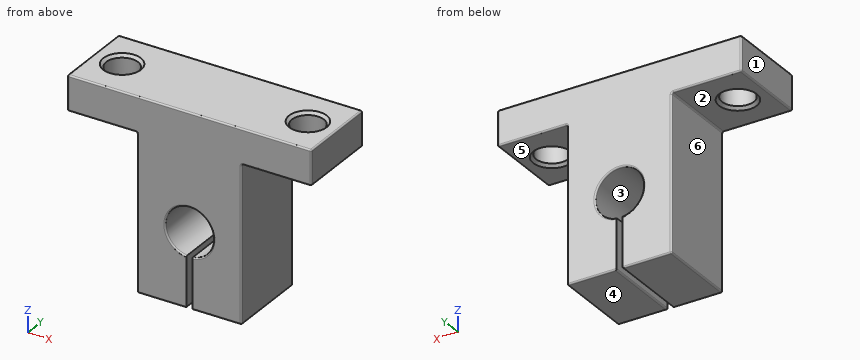
from build123d import *

# Parameters (mm, degrees)
BOSS_EXTRUDE1_DEPTH      = 7
BOSS_EXTRUDE1_DEPTH_BACK = 7
CUT_EXTRUDE1_REACH       = 34.8
SKETCH2_R                = 2.75
FILLET1_R                = 0.25
CHAMFER1_SIZE            = 0.5


with BuildPart() as part:
    # Sketch1 → Boss-Extrude1 (new body, two sides)
    with BuildSketch(Plane(origin=(0, 0, 0), x_dir=(1, 0, 0), z_dir=(0, 1, 0))) as boss_extrude1_sk:
        with BuildLine():
            Line((-21, 6), (-21, 0))
            Line((-21, 0), (0, 0))
            Line((0, 0), (0, 15.85))
            ThreePointArc((0, 15.85), (-4.142435459, 19.749543473), (-0.5, 24.119769411))
            Line((-0.5, 24.119769411), (-0.5, 32.8))
            Line((-0.5, 32.8), (-9, 32.8))
            Line((-9, 32.8), (-9, 6))
            Line((-9, 6), (-21, 6))
        make_face()
        with BuildLine():
            Line((0, 15.85), (0, 0))
            Line((0, 0), (21, 0))
            Line((21, 0), (21, 6))
            Line((21, 6), (9, 6))
            Line((9, 6), (9, 32.8))
            Line((9, 32.8), (0.5, 32.8))
            Line((0.5, 32.8), (0.5, 24.119769411))
            ThreePointArc((0.5, 24.119769411), (3.106243712, 22.752044694), (4.15, 20))
            ThreePointArc((4.15, 20), (2.934493142, 17.065506858), (0, 15.85))
        make_face()
    extrude(amount=BOSS_EXTRUDE1_DEPTH)
    extrude(boss_extrude1_sk.sketch, amount=-BOSS_EXTRUDE1_DEPTH_BACK)

    # Sketch2 → Cut-Extrude1 (cut, up to next)
    with BuildSketch(Plane.XY, mode=Mode.PRIVATE) as cut_extrude1_sk1:
        with Locations((-16, 0)):
            Circle(SKETCH2_R)
    cut_extrude1_tool1 = extrude(cut_extrude1_sk1.sketch, amount=-CUT_EXTRUDE1_REACH, mode=Mode.PRIVATE) & part.part
    add(cut_extrude1_tool1.solids().sort_by_distance((-16, 0, 0))[0], mode=Mode.SUBTRACT)
    # Sketch2 → Cut-Extrude1 (cut, up to next)
    with BuildSketch(Plane.XY, mode=Mode.PRIVATE) as cut_extrude1_sk2:
        with Locations((16, 0)):
            Circle(SKETCH2_R)
    cut_extrude1_tool2 = extrude(cut_extrude1_sk2.sketch, amount=-CUT_EXTRUDE1_REACH, mode=Mode.PRIVATE) & part.part
    add(cut_extrude1_tool2.solids().sort_by_distance((16, 0, 0))[0], mode=Mode.SUBTRACT)

    # Fillet1
    fillet1_edges = [part.edges().sort_by_distance(p)[0] for p in [
        (-4.75, -7, -32.8),
        (-9, -7, -19.4),
        (0.5, 0, -32.8),
        (9, 0, -32.8),
        (9, 0, -6),
        (21, 0, -6),
        (21, 0, 0),
        (-21, 0, 0),
        (-21, 0, -6),
        (-9, 0, -6),
        (-9, 0, -32.8),
        (-0.5, 0, -32.8),
        (-15, -7, -6),
        (-21, -7, -3),
        (0, 7, -15.85),
        (-4.75, 7, -32.8),
        (-21, 7, -3),
        (0, -7, 0),
        (15, 7, -6),
        (9, 7, -19.4),
        (4.75, 7, -32.8),
        (-9, 7, -19.4),
        (-15, 7, -6),
        (0, 7, 0),
        (21, 7, -3),
        (21, -7, -3),
        (15, -7, -6),
        (0, -7, -15.85),
        (9, -7, -19.4),
        (4.75, -7, -32.8),
    ]]
    fillet(fillet1_edges, radius=FILLET1_R)

    # Chamfer1
    chamfer1_edges = [part.edges().sort_by_distance(p)[0] for p in [
        (-18.75, 0, -6),
        (-18.75, 0, 0),
        (13.25, 0, 0),
        (13.25, 0, -6),
    ]]
    chamfer(chamfer1_edges, length=CHAMFER1_SIZE)


solid = part.part
Read the model definition and answer for the solid it produces. Units are mm, in the model's axes. Face numbers are marked on the shaded views. A direction names the side the tool comes from. Give positions to 0.01 mm unless a question says otherwise; leave off trailing zeros. Loops run counter-clockwise (first coordinate to the right, second up) from the corner with the lowest first, then second, coordinate; pieces in that order, holes last. Notation, with made-up numbers: M 64.5,35.5 L 96.5,35.5 A26 ccw 96.5,51.5 Z; hole C 41.25,20.25 d5. An arc over 180 degrees is marked long. Write each question's results on one line, items separated by ' | '.
1. Section A-A on x = -16 is taken. Give the vertices of the cut face in (y, z), plus the area to 3 significant figures.
Values:
outline: M -7,-5.75 A0.25 ccw -6.75,-6 L -3.25,-6 L -2.75,-5.5 L -2.75,-0.5 L -3.25,0 L -6.75,0 A0.25 ccw -7,-0.25 Z; M 2.75,-5.5 L 3.25,-6 L 6.75,-6 A0.25 ccw 7,-5.75 L 7,-0.25 A0.25 ccw 6.75,0 L 3.25,0 L 2.75,-0.5 Z | area: 50.4 mm^2
2. Section C-C on z = -15 is taken. Give the vertices of the cut face in (x, y), plus the area to 3 significant figures.
Values:
outline: M -9,-6.75 A0.25 ccw -8.75,-7 L 8.75,-7 A0.25 ccw 9,-6.75 L 9,6.75 A0.25 ccw 8.75,7 L -8.75,7 A0.25 ccw -9,6.75 Z | area: 252 mm^2
3. Section B-B on y = -5.5 is taken. Give the vertices of the cut face in (x, z).
Values:
outline: M -21,-5.75 A0.25 ccw -20.75,-6 L -9.25,-6 A0.25 cw -9,-6.25 L -9,-32.55 A0.25 ccw -8.75,-32.8 L -0.75,-32.8 A0.25 ccw -0.5,-32.55 L -0.5,-24.12 A4.15 cw long 0.5,-24.12 L 0.5,-32.55 A0.25 ccw 0.75,-32.8 L 8.75,-32.8 A0.25 ccw 9,-32.55 L 9,-6.25 A0.25 cw 9.25,-6 L 20.75,-6 A0.25 ccw 21,-5.75 L 21,-0.25 A0.25 ccw 20.75,0 L -20.75,0 A0.25 ccw -21,-0.25 Z
4. Given pin 1 (1 mm diameter, centred on y = -2.5, z = -19, fed in from +X); pin 2 (4 mm diameter, centred on y = 1.5, z = -28, fed in from -X); pin 3 (3.5 mm diameter, centred on x = -15, y = 1.5, fed in from -Z); pin 4 (6.5 mm diameter, centred on x = 0, z = -20, fed in from +Y), each flat-ended and moving along its own axis, determine where each tip first touches the part or whether it passes through.
Values:
pin 1: stops at x = 9 | pin 2: stops at x = -9 | pin 3: stops at z = -6 | pin 4: passes through
5. The mould has two halves that part along Z. Classify the marked faces 1, 2 and 3: pulls with the +Z half, pulls with the -Z half, needs draft (parallel to the pull), parting line crosses it, or undercut.
Values:
face 1: needs draft | face 2: pulls with the -Z half | face 3: undercut
6. Section D-D on x = -10 is taken. Give the vertices of the cut face in (y, z).
Values:
outline: M -7,-5.75 A0.25 ccw -6.75,-6 L 6.75,-6 A0.25 ccw 7,-5.75 L 7,-0.25 A0.25 ccw 6.75,0 L -6.75,0 A0.25 ccw -7,-0.25 Z
7. Straight lines are drawn through the part: line 1 (Y direction, x = -16, z = -4.2); line 2 (X direction, y = 1.75, z = -20); line 3 (X direction, y = -4.5, z = -14.5). For each, find the intervals that lie inside material, in ascending order. Write a range as [from, to].
Values:
line 1: y = [-7, -2.75], [2.75, 7] | line 2: x = [-9, -4.15], [4.15, 9] | line 3: x = [-9, 9]
8. A tool of negligible diameter and unlimited length cuts with its end or side. For the marked faces 4, 5 and 6, from which of +Z, -Z, +X, -X, +Y, -Y can it reach the whole face along a straight path? Write none if from no direction.
Values:
face 4: -Z, +X, -X, +Y, -Y | face 5: -Z, +X, +Y, -Y | face 6: -Z, -X, +Y, -Y
